from build123d import *

# Parameters (mm, degrees)
BOSS_EXTRU_1_DEPTH      = 107
ESQUISSE2_R             = 2.5
ENL_V_MAT_EXTRU_1_DEPTH = 108.537202865


with BuildPart() as part:
    # Esquisse1 → Boss.-Extru.1 (new, symmetric)
    with BuildSketch(Plane(origin=(0, 0, 0), x_dir=(0, 0, -1), z_dir=(1, 0, 0))):
        Polygon((-5, 9.5), (-4, 9.5), (-4, 1), (4, 1), (4, 9.5), (5, 9.5), (5, 0), (-5, 0), align=None)
    extrude(amount=BOSS_EXTRU_1_DEPTH, both=True)

    # Esquisse2 → Enlèv. mat.-Extru.1 (cut, through all)
    with BuildSketch(Plane.XZ):
        with Locations(Location((-88, 0, 0), (0, 0, 270))):
            Circle(ESQUISSE2_R)
        with Locations(Location((-79, 0, 0), (0, 0, 270))):
            Circle(ESQUISSE2_R)
        with Locations(Location((-70, 0, 0), (0, 0, 270))):
            Circle(ESQUISSE2_R)
        with Locations(Location((-56, 0, 0), (0, 0, 270))):
            Circle(ESQUISSE2_R)
        with Locations(Location((-47, 0, 0), (0, 0, 270))):
            Circle(ESQUISSE2_R)
        with Locations(Location((-38, 0, 0), (0, 0, 270))):
            Circle(ESQUISSE2_R)
        with Locations(Location((-24, 0, 0), (0, 0, 270))):
            Circle(ESQUISSE2_R)
        with Locations(Location((-15, 0, 0), (0, 0, 270))):
            Circle(ESQUISSE2_R)
        with Locations(Location((-6, 0, 0), (0, 0, 270))):
            Circle(ESQUISSE2_R)
        with Locations(Location((8, 0, 0), (0, 0, 270))):
            Circle(ESQUISSE2_R)
        with Locations(Location((17, 0, 0), (0, 0, 270))):
            Circle(ESQUISSE2_R)
        with Locations(Location((26, 0, 0), (0, 0, 270))):
            Circle(ESQUISSE2_R)
        with Locations(Location((40, 0, 0), (0, 0, 270))):
            Circle(ESQUISSE2_R)
        with Locations(Location((49, 0, 0), (0, 0, 270))):
            Circle(ESQUISSE2_R)
        with Locations(Location((58, 0, 0), (0, 0, 270))):
            Circle(ESQUISSE2_R)
        with Locations(Location((72, 0, 0), (0, 0, 270))):
            Circle(ESQUISSE2_R)
        with Locations(Location((81, 0, 0), (0, 0, 270))):
            Circle(ESQUISSE2_R)
        with Locations(Location((90, 0, 0), (0, 0, 270))):
            Circle(ESQUISSE2_R)
    extrude(amount=-ENL_V_MAT_EXTRU_1_DEPTH, mode=Mode.SUBTRACT)


solid = part.part
For this review, take the finished solid that the model builds, in its own axes (mm). A direction names the side the tool comes from. Round coordinates to 2 decimals unless told otherwise and drop trailing zeros. Write each loop counter-clockwise with the first axis right and the second up, starting at its lowest first coordinate (ties: lowest second). Pieces come first, ordered by that corner, then holes. Notation, with made-up numbers: (-31.5, 69.5) -> (-20.5, 69.5) arc R36 ccw to (-20.5, 104.5) -> close; hole circle Ø4 at (76, 34.25). An arc over 180 degrees is marked (long way). Put each result on its own line as item: value.
Q1. The part is to be moulded in two halves that separate along Z. For faces 1 (the cylindrical face through (92.48, 0.49, 0.33)), 2 (the flat face through (107, 0.5, 0.3)), 3 (the flat face through (1, 5, -5)), say which applies: released by +Z, released by -Z, zero draft, split by the parting line, or undercut.
Determined:
face 1: undercut
face 2: zero draft
face 3: released by -Z
Q2. Consider section B-B on y = 4.75. State the section outline as (x, z) points.
Determined:
outline: (-107, -5) -> (107, -5) -> (107, -4) -> (-107, -4) -> close; (-107, 4) -> (107, 4) -> (107, 5) -> (-107, 5) -> close
Q3. To check wall thickness, follow L1, parallel to Z at x = -60, y = 6.25; L2, parallel to Y at x = -63, z = 1; L3, parallel to Z at x = 49.5, y = 0.5. State the ranges of each line that lie inside material, in increasing order. Write a range as [from, to].
Determined:
L1: z = [-5, -4], [4, 5]
L2: y = [0, 1]
L3: z = [-5, -2.45], [2.45, 5]
Q4. Consider section C-C on x = 30.5. State the section outline as (y, z) points, and give its area (3 significant figures).
Determined:
outline: (0, -5) -> (9.5, -5) -> (9.5, -4) -> (1, -4) -> (1, 4) -> (9.5, 4) -> (9.5, 5) -> (0, 5) -> close
area: 27.0 mm^2
Q5. Clearance check with flat-ended pins moving along their axes: pin 1 Ø4 at (x, z) = (49, 0) entering from +Y; pin 2 Ø6 at (x, z) = (17, 0) entering from +Y. State where each tip first meets the part, or that it passes through.
Determined:
pin 1: passes through
pin 2: stops at y = 1
Q6. Machinability: for faces 4 (the flat face through (1, 0, 0)), 5 (the flat face through (1, 5, 4)), which of the approach directions +Z, -Z, +X, -X, +Y, -Y give a long, thin tool a straight path to every point of the face, cutting with its end or side? Answer none if there is none.
Determined:
face 4: +Z, -Z, +X, -X, -Y
face 5: +X, -X, +Y
Q7. Consider section A-A on x = -79. State the section outline as (y, z) points, and give its area (3 significant figures).
Determined:
outline: (0, -5) -> (9.5, -5) -> (9.5, -4) -> (1, -4) -> (1, -2.5) -> (0, -2.5) -> close; (0, 2.5) -> (1, 2.5) -> (1, 4) -> (9.5, 4) -> (9.5, 5) -> (0, 5) -> close
area: 22.0 mm^2
